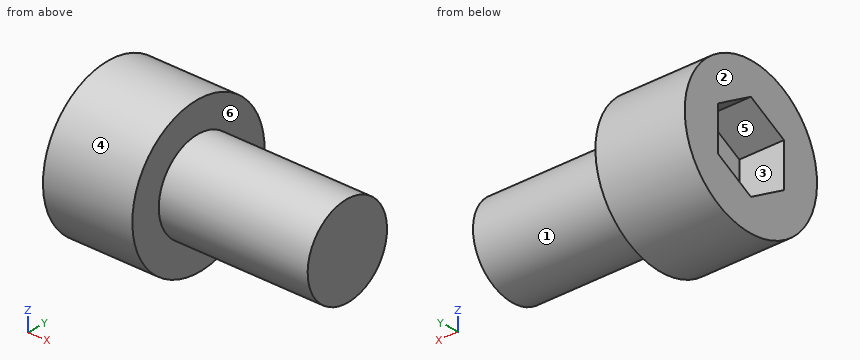
Solid Edge part; units mm, degrees
sketch "Sketch1" plane through (10.8674, 0, 10.8674) normal (0, -1, 0) x (1, 0, 0)
  line L0 (-18.8674, -10.8674) -> (-18.8674, -5.8674)
  line L1 (-18.8674, -5.8674) -> (-12.8674, -5.8674)
  line L2 (-12.8674, -5.8674) -> (-12.8674, -7.8674)
  line L3 (-12.8674, -7.8674) -> (-2.8674, -7.8674)
  line L4 (-2.8674, -7.8674) -> (-2.8674, -10.8674)
revolve "RevolvedProtrusion1" add sketch "Sketch1" angle 360 about axis through (16.5, 0, 0) along (-1, 0, 0)
sketch "Sketch2" plane through (-8, 0, 0) normal (-1, 0, 0) x (0, 0, -1)
  line L0 (2.8868, 0) -> (1.4434, 2.5)
  line L1 (1.4434, 2.5) -> (-1.4434, 2.5)
  line L2 (-1.4434, 2.5) -> (-2.8868, 0)
  line L3 (-2.8868, 0) -> (-1.4434, -2.5)
  line L4 (-1.4434, -2.5) -> (1.4434, -2.5)
  line L5 (1.4434, -2.5) -> (2.8868, 0)
extrude "Cutout1" cut sketch "Sketch2" against normal blind 3
cosmetic_thread "Gänga" thread depth 8
properties material "Steel"
The model under review builds one solid part; all positions refer to its coordinate system, in mm. Face numbers are marked on the shaded views. A direction names the side the tool comes from. Give positions to 0.01 mm unless a question says otherwise; leave off trailing zeros. Loops run counter-clockwise (first coordinate to the right, second up) from the corner with the lowest first, then second, coordinate; pieces in that order, holes last. Notation, with made-up numbers: (-5.75, 65) -> (52.25, 65) arc R34 cw to (52.25, 99) -> close; hole circle Ø4 at (34.5, 74). An arc over 180 degrees is marked (long way). Use CSV: the item, a comma, the result in double quotes.
1. Consider section B-B, the plane z = 0. Write out the cut boundary in (x, y).
Result:
outline,"(-8, -5) -> (-2, -5) -> (-2, -3) -> (8, -3) -> (8, 3) -> (-2, 3) -> (-2, 5) -> (-8, 5) -> (-8, 2.5) -> (-5, 2.5) -> (-5, -2.5) -> (-8, -2.5) -> close"
2. To check wall thickness, follow probe 1 along X at (y, z) = (-2.25, 0.5); probe 2 along X at (y, z) = (3.75, 2); probe 3 along Z at (x, y) = (-6.5, 4). State the ranges of each line that lie inside material, in increasing order. Write a range as from..to.
Result:
probe 1,"x = -5..8"
probe 2,"x = -8..-2"
probe 3,"z = -3..3"
3. Consider section A-A, the plane x = -5.5. Write out the cut boundary in (y, z).
Result:
outline,"circle Ø10 at (0, 0); hole (-2.5, -1.44) -> (0, -2.89) -> (2.5, -1.44) -> (2.5, 1.44) -> (0, 2.89) -> (-2.5, 1.44) -> close"
4. Consider section D-D, the plane x = 3.75. Write out the cut boundary in (y, z).
Result:
outline,"circle Ø6 at (0, 0)"
5. Consider section C-C, the plane y = 0.75. Write out the cut boundary in (x, z).
Result:
outline,"(-8, -4.94) -> (-2, -4.94) -> (-2, -2.9) -> (8, -2.9) -> (8, 2.9) -> (-2, 2.9) -> (-2, 4.94) -> (-8, 4.94) -> (-8, 2.45) -> (-5, 2.45) -> (-5, -2.45) -> (-8, -2.45) -> close"
6. For P1, Ø6, axis at x = -6, y = -3.5, coming from the -Z side; P2, Ø1, axis at x = 6.5, z = 2.5, coming from the -Y side; P3, Ø5, axis at x = 3, y = 0, coming from the -Z side, all flat-tipped, find the tip position at first contact; note any pin that passes through.
Result:
P1,"stops at z = -4.97"
P2,"stops at y = -2.24"
P3,"stops at z = -3"
7. Machinability: for the marked faces 4, 5 and 6, which of the approach directions +Z, -Z, +X, -X, +Y, -Y give a long, thin tool a straight path to every point of the face, cutting with its end or side? Answer none if there is none.
Result:
face 4,"+X, -X"
face 5,"-X"
face 6,"+X"
8. The part is to be moulded in two halves that separate along Z. For the marked faces 1, 2 and 3, say which applies: +Z half, -Z half, draft (parallel to the pull), parting line (faces both ways), or undercut.
Result:
face 1,"parting line"
face 2,"draft"
face 3,"undercut"
